Read the model definition and answer for the solid it produces. Units are mm, in the model's axes. Round coordinates to 2 decimals unless told otherwise and drop trailing zeros. Loops run counter-clockwise (first coordinate to the right, second up) from the corner with the lowest first, then second, coordinate; pieces in that order, holes last. Notation, with made-up numbers: (-32, -24) - (-7, -24) arc R26 ccw to (-7, -8) - close; hole circle Ø1 at (34, -2.75). An arc over 180 degrees is marked (long way). Answer as CSV lines item,"result".
```python
from build123d import *
from build123d.topology import SkipClean

# Parameters (mm, degrees)
EXTRUDE_1_DEPTH = 19
SKETCH_2_R      = 5
EXTRUDE_2_DEPTH = 16.2
SKETCH_5_W      = 1.1
SKETCH_5_H      = 0.2
EXTRUDE_START   = 176
SKETCH_4_R      = 5
EXTRUDE_4_DEPTH = 176
SKETCH_6_R      = 5
EXTRUDE_5_DEPTH = 26
EXTRUDE_START_2 = 26
SKETCH_7_R      = 5
EXTRUDE_6_DEPTH = 26


with BuildPart() as part:
    # Sketch 1 → Extrude 1 (new body)
    with BuildSketch(Plane(origin=(0, 0, 0), x_dir=(0, 0, -1), z_dir=(1, 0, 0))):
        with BuildLine():
            Line((-2.179449472, 4.5), (2.179449472, 4.5))
            ThreePointArc((2.179449472, 4.5), (0, -5), (-2.179449472, 4.5))
        make_face()
    extrude_1 = extrude(amount=EXTRUDE_1_DEPTH)

    # Sketch 2 → Extrude 2 (add)
    with BuildSketch(Plane(origin=(19, 0, 0), x_dir=(0, 0, -1), z_dir=(1, 0, 0))):
        with Locations(Location((0, 0, 0), (0, 0, 115.841932763))):
            Circle(SKETCH_2_R)
    extrude_2 = extrude(amount=EXTRUDE_2_DEPTH)

    # Sketch 5 → Cut-Revolve 1 (revolve, cut)
    with BuildSketch(Plane(origin=(0, 0, 0), x_dir=(1, 0, 0), z_dir=(0, 1, 0))):
        with Locations((31.95, 4.9)):
            Rectangle(SKETCH_5_W, SKETCH_5_H)
    cut_revolve_1 = revolve(axis=Axis((19, 0, 0), (-1, 0, 0)), mode=Mode.SUBTRACT)

    # Sketch 4 → Extrude 4 (add)
    with BuildSketch(Plane.ZY.offset(EXTRUDE_START)):
        Circle(SKETCH_4_R)
    extrude(amount=-EXTRUDE_4_DEPTH)

    # Mirror 1: Extrude 1, Extrude 2, Cut-Revolve 1 across plane
    add(extrude_1.mirror(Plane.ZY.offset(88)))
    add(extrude_2.mirror(Plane.ZY.offset(88)))
    add(cut_revolve_1.mirror(Plane.ZY.offset(88)), mode=Mode.SUBTRACT)

    # Sketch 6 → Extrude 5 (add)
    with SkipClean():  # the faces are left unmerged after this step: merging them gives an invalid solid
        with BuildSketch(Plane(origin=(35.2, 0, 0), x_dir=(0, 0, -1), z_dir=(1, 0, 0))):
            Circle(SKETCH_6_R)
        extrude(amount=EXTRUDE_5_DEPTH)

    # Sketch 7 → Extrude 6 (add)
    with SkipClean():  # the faces are left unmerged after this step: merging them gives an invalid solid
        with BuildSketch(Plane.ZY.offset(211.2).offset(EXTRUDE_START_2)):
            with Locations(Location((0, 0, 0), (0, 0, 180))):
                Circle(SKETCH_7_R)
        extrude(amount=-EXTRUDE_6_DEPTH)


solid = part.part
```
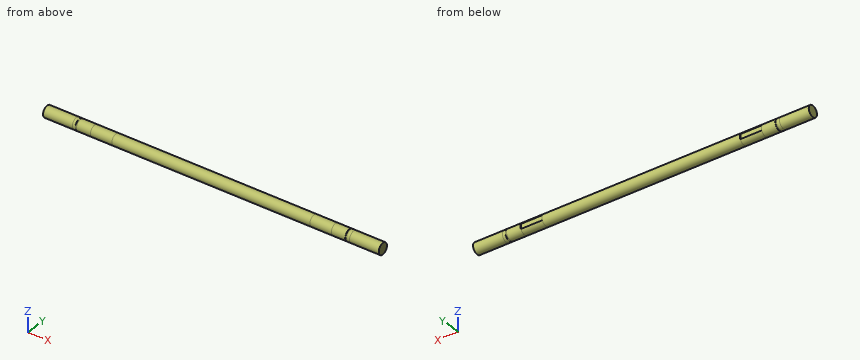
1) Each of these flat-tipped pins is pushed along its axis until it touches: P1, Ø2, axis at x = 14, z = 0, coming from the +Y side; P2, Ø3, axis at x = -201, y = 2, coming from the -Z side; P3, Ø3, axis at x = -122, y = -2.5, coming from the +Z side. Where does it stop, or does it pass through?
Entries:
P1,"stops at y = 4.5"
P2,"stops at z = -4.97"
P3,"stops at z = 4.9"
2) A cutting plane is placed at B-B, the plane x = -153.5. Determine the outline of the cut face in (y, z), plus the area to 3 significant figures.
Entries:
outline,"circle Ø10 at (0, 0)"
area,"78.5 mm^2"
3) Find the intervals of material crossed by line 1 (Y direction, x = -39.5, z = 3.75); line 2 (Y direction, x = -142.5, z = -0.75); line 3 (Z direction, x = -157, y = 1.5), in increasing order.
Entries:
line 1,"y = -3.31 to 3.31"
line 2,"y = -4.94 to 4.94"
line 3,"z = -4.77 to 4.77"
4) A cutting plane is placed at A-A, the plane y = -2.5. Determine the outline of the cut face in (x, z).
Entries:
outline,"(-237.2, -4.33) - (-208.5, -4.33) - (-208.5, -4.1) - (-207.4, -4.1) - (-207.4, -4.33) - (31.4, -4.33) - (31.4, -4.1) - (32.5, -4.1) - (32.5, -4.33) - (61.2, -4.33) - (61.2, 4.33) - (32.5, 4.33) - (32.5, 4.1) - (31.4, 4.1) - (31.4, 4.33) - (-207.4, 4.33) - (-207.4, 4.1) - (-208.5, 4.1) - (-208.5, 4.33) - (-237.2, 4.33) - close"
